Check sheet for the modelled part. Datum: model origin and axes. Units: mm. Coordinates: 2 decimals unless noted, no trailing zeros. Write each loop counter-clockwise with the first axis right and the second up, starting at its lowest first coordinate (ties: lowest second). Pieces come first, ordered by that corner, then holes. Notation, with made-up numbers: M 14,24.25 L 26,24.25 A27 cw 26,51.25 Z; hole C 10.25,8.5 d7. An arc over 180 degrees is marked long. Answer as CSV lines item,"result". Start each with the question number.
Q1. Mould release check, pull along X, two halves, no side actions. Record for faces 1 (the cylindrical face through (-29.09, -29.05, 1.01)), 2 (the cylindrical face through (27.88, 26.9, 0.99)), 3 (the flat face through (0, 0, 2)): pulls with the +X half, pulls with the -X half, needs draft (parallel to the pull), parting line crosses it, or undercut.
Q2. Sectioned sample at A-A, the plane x = -26. Record the cut outline in (y, z).
Q3. Depth check by flat-ended pin: pin 1 Ø2.5 at (x, y) = (-26.45, -26.45) entering from +Z. Enter the tip coordinate at first touch or a pass-through.
Q4. Thickness scan on line 1 along Y through (x, z) = (-26.45, 1.45); line 2 along X through (y, z) = (-27, 1.6); line 3 along X through (y, z) = (-26, 1.2). Record the ranges inside material, lowest first. Write a range as from..to.
from build123d import *

# Parameters (mm, degrees)
SKETCH1_W           = 59.9
SKETCH1_H           = 59.9
SKETCH1_R           = 1.5
BOSS_EXTRUDE1_DEPTH = 2
FILLET1_R           = 3


with BuildPart() as part:
    # Sketch1 → Boss-Extrude1 (new body)
    with BuildSketch(Plane.XY):
        Rectangle(SKETCH1_W, SKETCH1_H)
        with Locations((-26.45, -26.45)):
            Circle(SKETCH1_R, mode=Mode.SUBTRACT)
        with Locations((26.45, -26.45)):
            Circle(SKETCH1_R, mode=Mode.SUBTRACT)
        with Locations((-26.45, 26.45)):
            Circle(SKETCH1_R, mode=Mode.SUBTRACT)
        with Locations((26.45, 26.45)):
            Circle(SKETCH1_R, mode=Mode.SUBTRACT)
    extrude(amount=BOSS_EXTRUDE1_DEPTH)

    # Fillet1
    fillet1_edges = [part.edges().sort_by_distance(p)[0] for p in [
        (29.95, -29.95, 1),
        (-29.95, -29.95, 1),
        (-29.95, 29.95, 1),
        (29.95, 29.95, 1),
    ]]
    fillet(fillet1_edges, radius=FILLET1_R)


solid = part.part
Output:
1,face 1,"pulls with the -X half"
1,face 2,"undercut"
1,face 3,"needs draft"
2,outline,"M -29.95,0 L -27.88,0 L -27.88,2 L -29.95,2 Z; M -25.02,0 L 25.02,0 L 25.02,2 L -25.02,2 Z; M 27.88,0 L 29.95,0 L 29.95,2 L 27.88,2 Z"
3,pin 1,"passes through"
4,line 1,"y = -29.95..-27.95, -24.95..24.95, 27.95..29.95"
4,line 2,"x = -29.95..-27.85, -25.05..25.05, 27.85..29.95"
4,line 3,"x = -29.95..-27.88, -25.02..25.02, 27.88..29.95"
